from build123d import *

# Parameters (mm, degrees)
BASE_W                              = 36
BASE_H                              = 30
BOSS_EXTRUDE1_DEPTH                 = 4.5
WALLS_W                             = 36
WALLS_H                             = 5
WALLS_EXT_DEPTH                     = 31.5
SWITCH_BLOCK_W                      = 15
SWITCH_BLOCK_H                      = 30
SWITCH_BLOCK_EXT_DEPTH              = 15.25
MAGNET_POCKET_R                     = 6.25
MAGNET_POCKET_CUT_DEPTH             = 3.75
FILLET1_R                           = 5
FILLET2_R                           = 5
FILLET3_R                           = 20
FILLET4_R                           = 20
SWITCH_PLACE_W                      = 14
SWITCH_PLACE_H                      = 6
SWITCH_POCKET_DEPTH                 = 6.75
SWITCH_CONTACTS_W                   = 14
SWITCH_CONTACTS_H                   = 2.5
SWITCH_LEADS_DEPTH                  = 7
SWITCH_ANGLE_LEFT_DEPTH             = 1.75
SWITCH_ANGLE_RIGHT_DEPTH            = 1.75
WIRE_GUIDE_W                        = 8
WIRE_GUIDE_H                        = 4
WIRE_PASS_THROUGH_DEPTH             = 6
WIRE_PASS_THROUGH_DIRECTION_2_REACH = 39.071
WIRE_CHANNEL_OUTLINE_W              = 4
WIRE_CHANNEL_OUTLINE_H              = 4
WIRE_CHANNEL_DEPTH                  = 1.5
ACHSE_R                             = 1.1
M2_ACHSE_DEPTH                      = 55.002314765
M2_NUT_DEPTH                        = 2.5
SKETCH2_R                           = 1.575
M3_MOUNTING_SCREWS_DEPTH            = 4.5
SKETCH9_W                           = 2
SKETCH9_H                           = 1.5
BOSS_EXTRUDE3_DEPTH                 = 12
SKETCH10_W                          = 2
SKETCH10_H                          = 1.5
BOSS_EXTRUDE4_DEPTH                 = 12
SKETCH18_W                          = 8
SKETCH18_H                          = 11.5
BOSS_EXTRUDE5_DEPTH                 = 1
FILLET5_R                           = 1
FILLET6_R                           = 1
SKETCH19_W                          = 21
SKETCH19_H                          = 27
CUT_EXTRUDE1_DEPTH                  = 0.25
SKETCH20_W                          = 21
SKETCH20_H                          = 27
CUT_EXTRUDE2_DEPTH                  = 0.25
SKETCH21_R                          = 2
CUT_EXTRUDE3_DEPTH                  = 2


# Read off the part's stored shape, not the designer's step: Wire Channel
with BuildPart() as part:
    # Base → Boss-Extrude1 (new body)
    with BuildSketch(Plane(origin=(0, 0, 0), x_dir=(1, 0, 0), z_dir=(0, 1, 0))):
        Rectangle(BASE_W, BASE_H)
    extrude(amount=BOSS_EXTRUDE1_DEPTH)

    # Walls → Walls Ext (add)
    with BuildSketch(Plane.XZ):
        with Locations((0, 17.5)):
            Rectangle(WALLS_W, WALLS_H)
        with Locations((0, -17.5)):
            Rectangle(WALLS_W, WALLS_H)
    extrude(amount=-WALLS_EXT_DEPTH)

    # Switch Block → Switch Block Ext (add)
    with BuildSketch(Plane(origin=(0, 4.5, 0), x_dir=(1, 0, 0), z_dir=(0, 1, 0))):
        with Locations((-10.5, 0)):
            Rectangle(SWITCH_BLOCK_W, SWITCH_BLOCK_H)
    extrude(amount=SWITCH_BLOCK_EXT_DEPTH)

    # Magnet Pocket → Magnet Pocket Cut (cut)
    with BuildSketch(Plane(origin=(0, 0, 0), x_dir=(1, 0, 0), z_dir=(0, 1, 0))):
        with Locations(Location((10, 0, 0), (0, 0, 90))):
            Circle(MAGNET_POCKET_R)
    extrude(amount=MAGNET_POCKET_CUT_DEPTH, mode=Mode.SUBTRACT)

    # Fillet1
    fillet1_edges = [part.edges().sort_by_distance(p)[0] for p in [
        (-18, 31.5, -17.5),
    ]]
    fillet(fillet1_edges, radius=FILLET1_R)

    # Fillet2
    fillet2_edges = [part.edges().sort_by_distance(p)[0] for p in [
        (-18, 31.5, 17.5),
    ]]
    fillet(fillet2_edges, radius=FILLET2_R)

    # Fillet3
    fillet3_edges = [part.edges().sort_by_distance(p)[0] for p in [
        (18, 31.5, -17.5),
    ]]
    fillet(fillet3_edges, radius=FILLET3_R)

    # Fillet4
    fillet4_edges = [part.edges().sort_by_distance(p)[0] for p in [
        (18, 31.5, 17.5),
    ]]
    fillet(fillet4_edges, radius=FILLET4_R)

    # Switch Place → Switch Pocket (cut)
    with BuildSketch(Plane(origin=(0, 19.75, 0), x_dir=(1, 0, 0), z_dir=(0, 1, 0))):
        with Locations((-10, 0)):
            Rectangle(SWITCH_PLACE_W, SWITCH_PLACE_H)
    extrude(amount=-SWITCH_POCKET_DEPTH, mode=Mode.SUBTRACT)

    # Switch Contacts → Switch Leads (cut)
    with BuildSketch(Plane(origin=(0, 13, 0), x_dir=(1, 0, 0), z_dir=(0, 1, 0))):
        with Locations((-10, 0)):
            Rectangle(SWITCH_CONTACTS_W, SWITCH_CONTACTS_H)
    extrude(amount=-SWITCH_LEADS_DEPTH, mode=Mode.SUBTRACT)

    # Sketch16 → Switch Angle Left (add)
    with BuildSketch(Plane(origin=(0, 0, 3), x_dir=(-1, 0, 0), z_dir=(0, 0, -1))):
        Polygon((17, 13), (17, 13.75), (3, 13), align=None)
    extrude(amount=SWITCH_ANGLE_LEFT_DEPTH)

    # Sketch17 → Switch Angle Right (add)
    with BuildSketch(Plane.XY.offset(-3)):
        Polygon((-17, 13), (-17, 13.75), (-3, 13), align=None)
    extrude(amount=SWITCH_ANGLE_RIGHT_DEPTH)

    # Wire Guide → Wire pass through (cut)
    with BuildSketch(Plane(origin=(0, 6, 0), x_dir=(1, 0, 0), z_dir=(0, 1, 0))):
        with Locations((-10, 0)):
            Rectangle(WIRE_GUIDE_W, WIRE_GUIDE_H)
    extrude(amount=-WIRE_PASS_THROUGH_DEPTH, mode=Mode.SUBTRACT)

    # Wire pass through direction 2: up to this plane
    wire_pass_through_direction_2_end = Plane(origin=(-17, 13.75, -12.770074893), z_dir=(-0.05349472137161193, -0.9985681322700889, 0))
    # Wire Guide → Wire pass through direction 2 (cut, up to the surface)
    with BuildSketch(Plane(origin=(0, 6, 0), x_dir=(1, 0, 0), z_dir=(0, 1, 0)), mode=Mode.PRIVATE) as wire_pass_through_direction_2_sk1:
        with Locations((-10, 0)):
            Rectangle(WIRE_GUIDE_W, WIRE_GUIDE_H)
    wire_pass_through_direction_2_tool1 = split(extrude(wire_pass_through_direction_2_sk1.sketch, amount=WIRE_PASS_THROUGH_DIRECTION_2_REACH, mode=Mode.PRIVATE), bisect_by=wire_pass_through_direction_2_end, keep=Keep.BOTH, mode=Mode.PRIVATE)
    add(wire_pass_through_direction_2_tool1.solids().sort_by_distance((-10, 6, 0))[0], mode=Mode.SUBTRACT)

    # Wire Channel outline → Wire Channel (cut)
    with BuildSketch(Plane(origin=(0, 0, 0), x_dir=(1, 0, 0), z_dir=(0, 1, 0))):
        with Locations((-16, 0)):
            Rectangle(WIRE_CHANNEL_OUTLINE_W, WIRE_CHANNEL_OUTLINE_H)
        with BuildLine():
            Line((-6, 2), (-6, -2))
            Line((-6, -2), (0.968804066, -2))
            ThreePointArc((0.968804066, -2), (0.75, 0), (0.968804066, 2))
            Line((0.968804066, 2), (-6, 2))
        make_face()
    extrude(amount=WIRE_CHANNEL_DEPTH, mode=Mode.SUBTRACT)

    # Achse → M2 Achse (cut, through all)
    with BuildSketch(Plane.XY.offset(20)):
        with Locations((-10, 25.5)):
            Circle(ACHSE_R)
    extrude(amount=-M2_ACHSE_DEPTH, mode=Mode.SUBTRACT)

    # Sketch5 → M2 Nut (cut)
    with BuildSketch(Plane(origin=(0, 0, -20), x_dir=(-1, 0, 0), z_dir=(0, 0, -1))):
        Polygon((10, 27.6), (8.181346652, 26.55), (8.181346652, 24.45), (10, 23.4), (11.818653348, 24.45), (11.818653348, 26.55), align=None)
    extrude(amount=-M2_NUT_DEPTH, mode=Mode.SUBTRACT)

    # Sketch2 → M3 Mounting Screws (cut)
    with BuildSketch(Plane.XZ):
        with Locations(Location((2, -10, 0), (0, 0, 270))):
            Circle(SKETCH2_R)
        with Locations(Location((2, 10, 0), (0, 0, 270))):
            Circle(SKETCH2_R)
    extrude(amount=-M3_MOUNTING_SCREWS_DEPTH, mode=Mode.SUBTRACT)

    # M3 Senkkopf cone 1 section (through the dimple's axis) → M3 Senkkopf (revolve, cut)
    with BuildSketch(Plane(origin=(2, 4.5, 10), x_dir=(0, 0, 1), z_dir=(1, 0, 0))):
        Polygon((0, 0), (3.25, 0), (0, 3.25), align=None)
    revolve(axis=Axis((2, 4.5, 10), (0, -1, 0)), mode=Mode.SUBTRACT)

    # M3 Senkkopf cone 2 section (through the dimple's axis) → M3 Senkkopf cone 2 (revolve, cut)
    with BuildSketch(Plane(origin=(2, 4.5, -10), x_dir=(0, 0, 1), z_dir=(1, 0, 0))):
        Polygon((0, 0), (3.25, 0), (0, 3.25), align=None)
    revolve(axis=Axis((2, 4.5, -10), (0, -1, 0)), mode=Mode.SUBTRACT)

    # Sketch9 → Boss-Extrude3 (add)
    with BuildSketch(Plane.XY.offset(-15)):
        with Locations((-17, 20.5)):
            Rectangle(SKETCH9_W, SKETCH9_H)
    extrude(amount=BOSS_EXTRUDE3_DEPTH)

    # Sketch10 → Boss-Extrude4 (add)
    with BuildSketch(Plane(origin=(0, 0, 15), x_dir=(-1, 0, 0), z_dir=(0, 0, -1))):
        with Locations((17, 20.5)):
            Rectangle(SKETCH10_W, SKETCH10_H)
    extrude(amount=BOSS_EXTRUDE4_DEPTH)

    # Sketch18 → Boss-Extrude5 (add)
    with BuildSketch(Plane(origin=(-3, 0, 0), x_dir=(0, 0, -1), z_dir=(1, 0, 0))):
        with Locations((0, 10.25)):
            Rectangle(SKETCH18_W, SKETCH18_H)
    extrude(amount=BOSS_EXTRUDE5_DEPTH)

    # Fillet5
    fillet5_edges = [part.edges().sort_by_distance(p)[0] for p in [
        (-2, 10.25, 4),
    ]]
    fillet(fillet5_edges, radius=FILLET5_R - 0.0001)  # a hair under: the kernel refuses the full size

    # Fillet6
    fillet6_edges = [part.edges().sort_by_distance(p)[0] for p in [
        (-2, 10.25, -4),
    ]]
    fillet(fillet6_edges, radius=FILLET6_R - 0.0001)  # a hair under: the kernel refuses the full size

    # Sketch19 → Cut-Extrude1 (cut)
    with BuildSketch(Plane(origin=(0, 0, 15), x_dir=(-1, 0, 0), z_dir=(0, 0, -1))):
        with Locations((-7.5, 18)):
            Rectangle(SKETCH19_W, SKETCH19_H)
    extrude(amount=-CUT_EXTRUDE1_DEPTH, mode=Mode.SUBTRACT)

    # Sketch20 → Cut-Extrude2 (cut)
    with BuildSketch(Plane.XY.offset(-15)):
        with Locations((7.5, 18)):
            Rectangle(SKETCH20_W, SKETCH20_H)
    extrude(amount=-CUT_EXTRUDE2_DEPTH, mode=Mode.SUBTRACT)

    # Sketch21 → Cut-Extrude3 (cut)
    with BuildSketch(Plane.XY.offset(20)):
        with Locations((-10, 25.5)):
            Circle(SKETCH21_R)
    extrude(amount=-CUT_EXTRUDE3_DEPTH, mode=Mode.SUBTRACT)


solid = part.part
Can you work these out from the model? Positions are in its coordinate system, mm. A direction names the side the tool comes from. Coordinates: 2 decimals unless noted, no trailing zeros. Loops run counter-clockwise (first coordinate to the right, second up) from the corner with the lowest first, then second, coordinate; pieces in that order, holes last. Notation, with made-up numbers: (52, 27) - (77, 27) arc R20 cw to (77, 49) - close; hole circle Ø11 at (39.5, 19.25). An arc over 180 degrees is marked (long way). Answer as a JSON object with one key per item and string values. Group by question number.
Item 1: If we section it at D-D (y = 25.5): List the corners of the cut face in (x, z) for me.
Item 2: For pin 1 (8 mm diameter, centred on y = 23, z = 9, fed in from +X); pin 2 (3.5 mm diameter, centred on x = -10, y = 25.5, fed in from +Z); pin 3 (6.5 mm diameter, centred on y = 14, z = -1.5, fed in from +X), each with a flat end and sliding along its axis, tell me the tip position at first contact or that it passes through.
Item 3: On a 3-axis mill with a long thin cutter (end or side, diameter ignored), from which of +Z, -Z, +X, -X, +Y, -Y can I reach the whole of each face in a straight line? I mean faces 4 (the face through (-14, 5, 0)), 5 (the face through (-5, 6, 0)), 6 (the face through (-3, 12, -9)). Say none if no direction works.
Item 4: If we mould it in two halves opening along X, with no side actions, what happens to faces 1 (the face through (-8, 31.5, -17)), 2 (the face through (-9, 7, 2)), 3 (the face through (18, 3, 0))? For each: released by +X, released by -X, zero draft, split by the parting line, or undercut.
Item 5: If I drill on L1, parallel to Z at x = 2, y = 1.8 (3 decimals); L2, parallel to Z at x = 2.5, y = 23; L3, parallel to Z at x = -3.5, y = 9.5, over which ranges is the centre line in solid material (lowest first)? Write a range as from..to.
Item 6: If we section it at A-A (z = 0): List the corners of the cut face in (x, y) for me.
Item 7: If we section it at C-C (z = -17): List the corners of the cut face in (x, y) for me.
Returned:
{
 "1": {"outline": "(-18, -20) - (-11.82, -20) - (-11.82, -17.5) - (-11.1, -17.5) - (-11.1, -15) - (-18, -15) - close; (-18, 15) - (-11.1, 15) - (-11.1, 18) - (-12, 18) - (-12, 20) - (-18, 20) - close; (-8.9, -17.5) - (-8.18, -17.5) - (-8.18, -20) - (12.28, -20) - (12.28, -15.25) - (-3, -15.25) - (-3, -15) - (-8.9, -15) - close; (-8.9, 15) - (-3, 15) - (-3, 15.25) - (12.28, 15.25) - (12.28, 20) - (-8, 20) - (-8, 18) - (-8.9, 18) - close"},
 "2": {"pin 1": "stops at x = -3", "pin 2": "stops at z = 18", "pin 3": "stops at x = -2"},
 "3": {"face 4": "+Y, -Y", "face 5": "+Y", "face 6": "+X, +Y"},
 "4": {"face 1": "zero draft", "face 2": "undercut", "face 3": "released by +X"},
 "5": {"L1": "z = -20..-11.575, -8.425..8.425, 11.575..20", "L2": "z = -20..-15.25, 15.25..20", "L3": "z = -20..-1.25, 1.25..20"},
 "6": {"outline": "(-18, 1.5) - (-14, 1.5) - (-14, 6) - (-17, 6) - (-17, 19.75) - (-18, 19.75) - close; (-6, 1.5) - (0.75, 1.5) - (0.75, 0) - (3.75, 0) - (3.75, 3.75) - (16.25, 3.75) - (16.25, 0) - (18, 0) - (18, 4.5) - (-2, 4.5) - (-2, 16) - (-3, 16) - (-3, 6) - (-6, 6) - close"},
 "7": {"outline": "(-18, 0) - (18, 0) - (18, 11.5) arc R20 ccw to (-2, 31.5) - (-13, 31.5) arc R5 ccw to (-18, 26.5) - close; hole circle Ø2.2 at (-10, 25.5)"}
}
